Build history of the part. All positions in model axes, mm. Coordinates: 2 decimals unless noted, no trailing zeros. Write each loop counter-clockwise with the first axis right and the second up, starting at its lowest first coordinate (ties: lowest second). Pieces come first, ordered by that corner, then holes.
from build123d import *

# Parameters (mm, degrees)
SKETCH1_R           = 30
BOSS_EXTRUDE1_DEPTH = 5
CHAMFER1_SIZE       = 0.4


# Read off the part's stored shape, not the designer's step: CSK for M3 Hex Socket Countersunk Cap Screw1
with BuildPart() as part:
    # Sketch1 → Boss-Extrude1 (new body)
    with BuildSketch(Plane(origin=(0, 0, 0), x_dir=(1, 0, 0), z_dir=(0, 1, 0))):
        with Locations(Location((0, 0, 0), (0, 0, 270))):
            Circle(SKETCH1_R)
    extrude(amount=BOSS_EXTRUDE1_DEPTH)

    # CSK for M3 Hex Socket Countersunk Ca 2 → CSK for M3 Hex Socket Countersunk Cap Screw1 (revolve, cut)
    with BuildSketch(Plane(origin=(8, 0, 13.856406461), x_dir=(1, 0, 0), z_dir=(0, 0, 1))):
        Polygon((0, 0), (1.8, 0), (1.8, 3.44), (3.36, 5), (0, 5), align=None)
    revolve(axis=Axis((8, 0, 13.856406461), (0, 1, 0)), mode=Mode.SUBTRACT)

    # CSK for M3 Hex Socket Countersunk Ca 3 o → CSK for M3 Hex Socket Countersunk Ca 3 (revolve, cut)
    with BuildSketch(Plane(origin=(-8, 0, 13.856406461), x_dir=(1, 0, 0), z_dir=(0, 0, 1))):
        Polygon((0, 0), (1.8, 0), (1.8, 3.44), (3.36, 5), (0, 5), align=None)
    revolve(axis=Axis((-8, 0, 13.856406461), (0, 1, 0)), mode=Mode.SUBTRACT)

    # CSK for M3 Hex Socket Countersunk Ca 4 o → CSK for M3 Hex Socket Countersunk Ca 4 (revolve, cut)
    with BuildSketch(Plane(origin=(-16, 0, 0), x_dir=(1, 0, 0), z_dir=(0, 0, 1))):
        Polygon((0, 0), (1.8, 0), (1.8, 3.44), (3.36, 5), (0, 5), align=None)
    revolve(axis=Axis((-16, 0, 0), (0, 1, 0)), mode=Mode.SUBTRACT)

    # CSK for M3 Hex Socket Countersunk Ca 5 o → CSK for M3 Hex Socket Countersunk Ca 5 (revolve, cut)
    with BuildSketch(Plane(origin=(-8, 0, -13.856406461), x_dir=(1, 0, 0), z_dir=(0, 0, 1))):
        Polygon((0, 0), (1.8, 0), (1.8, 3.44), (3.36, 5), (0, 5), align=None)
    revolve(axis=Axis((-8, 0, -13.856406461), (0, 1, 0)), mode=Mode.SUBTRACT)

    # CSK for M3 Hex Socket Countersunk Ca 6 o → CSK for M3 Hex Socket Countersunk Ca 6 (revolve, cut)
    with BuildSketch(Plane(origin=(8, 0, -13.856406461), x_dir=(1, 0, 0), z_dir=(0, 0, 1))):
        Polygon((0, 0), (1.8, 0), (1.8, 3.44), (3.36, 5), (0, 5), align=None)
    revolve(axis=Axis((8, 0, -13.856406461), (0, 1, 0)), mode=Mode.SUBTRACT)

    # CSK for M3 Hex Socket Countersunk Ca 7 o → CSK for M3 Hex Socket Countersunk Ca 7 (revolve, cut)
    with BuildSketch(Plane(origin=(16, 0, 0), x_dir=(1, 0, 0), z_dir=(0, 0, 1))):
        Polygon((0, 0), (1.8, 0), (1.8, 3.44), (3.36, 5), (0, 5), align=None)
    revolve(axis=Axis((16, 0, 0), (0, 1, 0)), mode=Mode.SUBTRACT)

    # Chamfer1
    chamfer1_edges = [part.edges().sort_by_distance(p)[0] for p in [
        (0, 5, -30),
    ]]
    chamfer(chamfer1_edges, length=CHAMFER1_SIZE)


solid = part.part
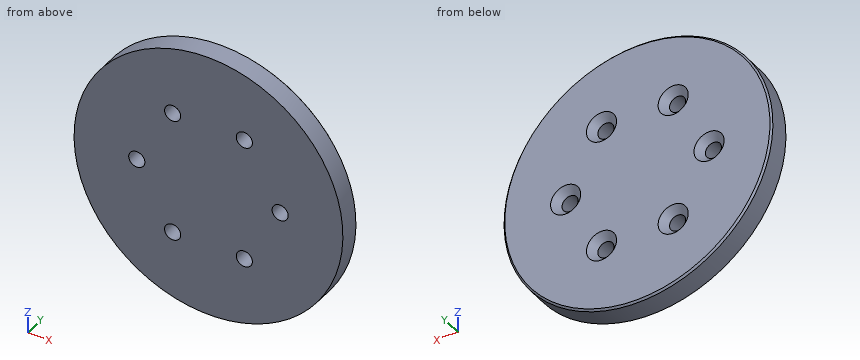
(1) Slice it at A-A, the plane z = 0. List the corners of the cut face in (x, y), and give its area (3 significant figures).
(2) Slice it at B-B, the plane x = 8. Give the number of separate pieces and of enclosed holes in the cut face, and give its area (3 significant figures).
(3) Flat gauge pins, fed straight in: P1, Ø3, axis at x = -21.5, y = 3, coming from the -Z side; P2, Ø1.5, axis at x = -11.5, y = 4.5, coming from the +Z side; P3, Ø4.5, axis at x = 16, z = 0, coming from the +Y side. Where does each tip first touch, or does it go through?
(4) Probe L1, parallel to X at y = 2.3, z = 0; L2, parallel to Z at x = -8, y = 1.2; L3, parallel to Z at x = -17.5, y = 3.3. List the from-to ranges inside material, lowest first.
Results:
1. outline: (-30, 0) - (-17.8, 0) - (-17.8, 3.44) - (-19.36, 5) - (-29.6, 5) - (-30, 4.6) - close; (-14.2, 0) - (14.2, 0) - (14.2, 3.44) - (12.64, 5) - (-12.64, 5) - (-14.2, 3.44) - close; (17.8, 0) - (30, 0) - (30, 4.6) - (29.6, 5) - (19.36, 5) - (17.8, 3.44) - close
1. area: 259 mm2
2. separate pieces: 3
2. enclosed holes: 0
2. area: 248 mm2
3. P1: stops at z = -22.36
3. P2: stops at z = 28.01
3. P3: stops at y = 3.89
4. L1: x = -30 to -17.8, -14.2 to 14.2, 17.8 to 30
4. L2: z = -28.91 to -15.66, -12.06 to 12.06, 15.66 to 28.91
4. L3: z = -24.37 to -0.99, 0.99 to 24.37
